from build123d import *

# Parameters (mm, degrees)
BASES_W                            = 14
BASES_H                            = 14
BASE_DEPTH                         = 14.5
NEUTRALS_W                         = 0.5
NEUTRALS_H                         = 2.8
NEUTRAL_DEPTH                      = 18.557049866
GROUNDS_W                          = 2.8
GROUNDS_H                          = 0.5
GROUND_DEPTH                       = 18.557049866
TOP_GROUND_AREA_REACH              = 23.337
SKETCH1_W                          = 2.8
SKETCH1_H                          = 11.5
SKETCH15_W                         = 2.8
SKETCH15_H                         = 12.5
GND_POCKET_EXTRA_CUT_DEPTH         = 1.75
SIDE_GROUND_AREA_DEPTH             = 5
SIDE_GND_TERMINAL_SCREW_AREA_REACH = 23.337
POCKET_START                       = -1.75
SKETCH4_W                          = 7.4
SKETCH4_H                          = 4
POCKET_GND_TERMINAL_AREA_DEPTH     = 2
SKETCH6_W                          = 12.5
SKETCH6_H                          = 3.6
NEUTRAL_SIDE_AREA_CUT_DEPTH        = 4.35
NEUTRAL_SIDE_SCREW_TERMINAL_DEPTH  = 8.4
NEUTRAL_SIDE_CURVED_WALL_CUT_REACH = 19.557
SKETCH8_W                          = 12.5
SKETCH8_H                          = 2.8
LINE_AREA_CUT_DEPTH                = 4.35
LINE_SIDE_SCREW_TERMINAL_REACH     = 23.337
SKETCH10_W                         = 7
SKETCH10_H                         = 12.3
BOTTOM_POCKET_DEPTH                = 4
SKETCH11_R                         = 2.5
FASTENER_TOP_BORE_DEPTH            = 0.5
SKETCH13_R                         = 2.35
FASTENER_BOSS_DEPTH                = 6.4
FASTENER_BOSS_TAPER                = 1
SKETCH12_R                         = 2
SKETCH14_R                         = 1.638287584


with BuildPart() as part:
    # BaseS → BASE (new body)
    with BuildSketch(Plane.XY):
        Rectangle(BASES_W, BASES_H)
    extrude(amount=BASE_DEPTH)

    # NeutralS → NEUTRAL (cut, through all)
    with BuildSketch(Plane(origin=(0, 0, 0), x_dir=(-1, 0, 0), z_dir=(0, 0, -1))):
        with Locations((4.65, 0)):
            Rectangle(NEUTRALS_W, NEUTRALS_H)
    neutral = extrude(amount=-NEUTRAL_DEPTH, mode=Mode.SUBTRACT)

    # LINE HM: NEUTRAL across plane
    add(neutral.mirror(Plane(origin=(0, 0, 0), x_dir=(0, 0, 1), z_dir=(1, 0, 0))), mode=Mode.SUBTRACT)

    # GroundS → GROUND (cut, through all)
    with BuildSketch(Plane(origin=(0, 0, 0), x_dir=(-1, 0, 0), z_dir=(0, 0, -1))):
        with Locations((0, 4.55)):
            Rectangle(GROUNDS_W, GROUNDS_H)
    extrude(amount=-GROUND_DEPTH, mode=Mode.SUBTRACT)

    # Sketch1 → TOP GROUND AREA (cut, up to next)
    with BuildSketch(Plane(origin=(0, 7, 0), x_dir=(1, 0, 0), z_dir=(0, 1, 0)), mode=Mode.PRIVATE) as top_ground_area_sk1:
        with Locations((0, -7.75)):
            Rectangle(SKETCH1_W, SKETCH1_H)
    top_ground_area_tool1 = extrude(top_ground_area_sk1.sketch, amount=-TOP_GROUND_AREA_REACH, mode=Mode.PRIVATE) & part.part
    add(top_ground_area_tool1.solids().sort_by_distance((0, 7, 7.75))[0], mode=Mode.SUBTRACT)

    # Sketch15 → GND POCKET EXTRA CUT (cut)
    with BuildSketch(Plane(origin=(0, 4.3, 0), x_dir=(1, 0, 0), z_dir=(0, 1, 0))):
        with Locations((0, -8.25)):
            Rectangle(SKETCH15_W, SKETCH15_H)
    extrude(amount=-GND_POCKET_EXTRA_CUT_DEPTH, mode=Mode.SUBTRACT)

    # Sketch2 → SIDE GROUND AREA (cut)
    with BuildSketch(Plane.XY.offset(14.5)):
        with BuildLine():
            Line((4, 7), (4, 4.05))
            ThreePointArc((4, 4.05), (3.707106781, 3.342893219), (3, 3.05))
            Line((3, 3.05), (0.6, 3.05))
            Line((0.6, 3.05), (0.6, 2.55))
            Line((0.6, 2.55), (-1.4, 2.55))
            Line((-1.4, 2.55), (-1.4, 7))
            Line((-1.4, 7), (4, 7))
        make_face()
    extrude(amount=-SIDE_GROUND_AREA_DEPTH, mode=Mode.SUBTRACT)

    # SIDE GND TERMINAL SCREW AREA: up to this face of the body (flat: up to its plane)
    side_gnd_terminal_screw_area_end = Plane(part.part.faces().sort_by_distance((1.4, 4.635, 6.044915254))[0])
    # Sketch3 → SIDE GND TERMINAL SCREW AREA (cut, up to the picked face)
    with BuildSketch(Plane(origin=(7, 0, 0), x_dir=(0, 0, -1), z_dir=(1, 0, 0)), mode=Mode.PRIVATE) as side_gnd_terminal_screw_area_sk1:
        with BuildLine():
            Line((-9.5, 9.45), (-9.5, 4.55))
            ThreePointArc((-9.5, 4.55), (-11.5, 2.55), (-13.5, 4.55))
            Line((-13.5, 4.55), (-13.5, 9.45))
            ThreePointArc((-13.5, 9.45), (-11.5, 11.45), (-9.5, 9.45))
        make_face()
    side_gnd_terminal_screw_area_tool1 = split(extrude(side_gnd_terminal_screw_area_sk1.sketch, amount=-SIDE_GND_TERMINAL_SCREW_AREA_REACH, mode=Mode.PRIVATE), bisect_by=side_gnd_terminal_screw_area_end, keep=Keep.BOTH, mode=Mode.PRIVATE)
    add(side_gnd_terminal_screw_area_tool1.solids().sort_by(Axis((7, 7, 11.5), (-1, 0, 0)))[0], mode=Mode.SUBTRACT)

    # Sketch4 → POCKET GND TERMINAL AREA (cut)
    with BuildSketch(Plane(origin=(0, 4.3, 0), x_dir=(1, 0, 0), z_dir=(0, 1, 0)).offset(POCKET_START)):
        with Locations((2.3, -11.5)):
            Rectangle(SKETCH4_W, SKETCH4_H)
    extrude(amount=POCKET_GND_TERMINAL_AREA_DEPTH, mode=Mode.SUBTRACT)

    # Sketch6 → NEUTRAL SIDE AREA CUT (cut)
    with BuildSketch(Plane.ZY.offset(7)):
        with Locations((8.25, 0.4)):
            Rectangle(SKETCH6_W, SKETCH6_H)
    extrude(amount=-NEUTRAL_SIDE_AREA_CUT_DEPTH, mode=Mode.SUBTRACT)

    # Sketch5 → NEUTRAL SIDE SCREW TERMINAL (cut)
    with BuildSketch(Plane(origin=(0, 7, 0), x_dir=(1, 0, 0), z_dir=(0, 1, 0))):
        with BuildLine():
            Line((-9.35, -9.5), (-4.65, -9.5))
            ThreePointArc((-4.65, -9.5), (-2.65, -11.5), (-4.65, -13.5))
            Line((-4.65, -13.5), (-9.35, -13.5))
            ThreePointArc((-9.35, -13.5), (-11.35, -11.5), (-9.35, -9.5))
        make_face()
    extrude(amount=-NEUTRAL_SIDE_SCREW_TERMINAL_DEPTH, mode=Mode.SUBTRACT)

    # Sketch7 → NEUTRAL SIDE CURVED WALL CUT (cut, up to next)
    with BuildSketch(Plane.XY.offset(14.5), mode=Mode.PRIVATE) as neutral_side_curved_wall_cut_sk1:
        with BuildLine():
            Line((-7, 2.2), (-2.65, 2.2))
            Line((-2.65, 2.2), (-2.65, 3))
            ThreePointArc((-2.65, 3), (-2.942893219, 3.707106781), (-3.65, 4))
            Line((-3.65, 4), (-7, 4))
            Line((-7, 4), (-7, 2.2))
        make_face()
    neutral_side_curved_wall_cut_tool1 = extrude(neutral_side_curved_wall_cut_sk1.sketch, amount=-NEUTRAL_SIDE_CURVED_WALL_CUT_REACH, mode=Mode.PRIVATE) & part.part
    add(neutral_side_curved_wall_cut_tool1.solids().sort_by_distance((-4.879997, 3.080933, 14.5))[0], mode=Mode.SUBTRACT)

    # Sketch8 → LINE AREA CUT (cut)
    with BuildSketch(Plane(origin=(7, 0, 0), x_dir=(0, 0, -1), z_dir=(1, 0, 0))):
        with Locations((-8.25, 0)):
            Rectangle(SKETCH8_W, SKETCH8_H)
    extrude(amount=-LINE_AREA_CUT_DEPTH, mode=Mode.SUBTRACT)

    # Sketch9 → LINE SIDE SCREW TERMINAL (cut, up to next)
    with BuildSketch(Plane(origin=(0, -7, 0), x_dir=(-1, 0, 0), z_dir=(0, -1, 0)), mode=Mode.PRIVATE) as line_side_screw_terminal_sk1:
        with BuildLine():
            Line((-4.65, -13.5), (-7, -13.5))
            ThreePointArc((-7, -13.5), (-9, -11.5), (-7, -9.5))
            Line((-7, -9.5), (-4.65, -9.5))
            ThreePointArc((-4.65, -9.5), (-2.65, -11.5), (-4.65, -13.5))
        make_face()
    line_side_screw_terminal_tool1 = extrude(line_side_screw_terminal_sk1.sketch, amount=-LINE_SIDE_SCREW_TERMINAL_REACH, mode=Mode.PRIVATE) & part.part
    add(line_side_screw_terminal_tool1.solids().sort_by_distance((5.825, -7, 11.5))[0], mode=Mode.SUBTRACT)

    # Sketch10 → BOTTOM POCKET (cut)
    with BuildSketch(Plane.XZ.offset(7)):
        with Locations((-1.5, 8.35)):
            Rectangle(SKETCH10_W, SKETCH10_H)
    extrude(amount=-BOTTOM_POCKET_DEPTH, mode=Mode.SUBTRACT)

    # Sketch11 → FASTENER TOP BORE (cut)
    with BuildSketch(Plane(origin=(0, 0, 0), x_dir=(-1, 0, 0), z_dir=(0, 0, -1))):
        Circle(SKETCH11_R)
    extrude(amount=-FASTENER_TOP_BORE_DEPTH, mode=Mode.SUBTRACT)

    # Sketch13 → FASTENER BOSS (add)
    with BuildSketch(Plane.XY.offset(14.5)):
        Circle(SKETCH13_R)
    extrude(amount=FASTENER_BOSS_DEPTH, taper=FASTENER_BOSS_TAPER)

    # Sketch12 → FASTENER CLEARANCE HOLE section 0
    with BuildSketch(Plane(origin=(0, 0, 0.5), x_dir=(-1, 0, 0), z_dir=(0, 0, -1))):
        Circle(SKETCH12_R)
    # Sketch14 → FASTENER CLEARANCE HOLE section 1
    with BuildSketch(Plane.XY.offset(20.9)):
        Circle(SKETCH14_R)
    loft(mode=Mode.SUBTRACT)


solid = part.part
Build history of the part. All positions in model axes, mm. A direction names the side the tool comes from. Round coordinates to 2 decimals unless told otherwise and drop trailing zeros. Order: outer loops, then holes, each group sorted by start corner. A loop starts at its lowest first (then second) coordinate and runs counter-clockwise, first axis right, second up. Notation, with made-up numbers: M -27,62 L 14,62 A29 cw 14,97 Z; hole C 51.5,43.5 d4. An arc over 180 degrees is marked long. Use CSV: the item, a comma, the result in double quotes. Start each with the question number.
(1) Cut at A-A on x = 6.25. List the corners of the cut face in (y, z), then the cut area to 3 significant figures.
(2) Flat gauge pins, fed straight in: P1, Ø0.5, axis at x = 3.5, y = 0.5, coming from the +Z side; P2, Ø4.5, axis at x = -1.5, y = -4.5, coming from the +Z side; P3, Ø1.5, axis at x = -2, z = 18, coming from the -Y side. Where does each tip first touch, or does it go through?
(3) Cut at B-B on y = -4.25. List the corners of the cut face in (x, z).
(4) Cut at C-C on z = 8.5. List the corners of the cut face in (x, y).
(5) Mould opens along X. For faces 5 (the face through (-4.4, 0, 1)), 6 (the face through (4, 0, 2)), 7 (the face through (2.65, -4.24, 11.46)) say: +X half, -X half, draft (parallel to the pull), parting line (faces both ways), or undercut.
(6) Tool access for faces 1 (the face through (6.51, 2.55, 11.46)), 2 (the face through (6, 0, 2)), 3 (the face through (0, 4.3, 1)), 4 (the face through (-2, -3, 8)): list every direction of +Z, -Z, +X, -X, +Y, -Y with a clear straight run to the whole face (end or side of a thin tool).
(7) Drill centre lines: probe 1 along Y at (x, z) = (0, 0.35); probe 2 along Z at (x, y) = (4.75, 4.75); probe 3 along Y at (x, z) = (3, 6.25). Where is each one in solid material? Low to high.
(8) Cut at D-D on x = -4. List the corners of the cut face in (y, z).
Findings:
1,outline,"M -7,0 L 7,0 L 7,9.5 L 4.55,9.5 A2 cw 4.55,13.5 L 7,13.5 L 7,14.5 L 1.4,14.5 L 1.4,2 L -1.4,2 L -1.4,9.5 L -7,9.5 Z; M -7,13.5 L -1.4,13.5 L -1.4,14.5 L -7,14.5 Z"
1,area,"130 mm^2"
2,P1,"stops at z = 2"
2,P2,"stops at z = 14.5"
2,P3,"stops at y = -1.92"
3,outline,"M -7,0 L 7,0 L 7,9.5 L 4.65,9.5 A2 cw 4.65,13.5 L 7,13.5 L 7,14.5 L 2,14.5 L 2,2.2 L -5,2.2 L -5,14.5 L -7,14.5 Z"
4,outline,"M -7,-7 L -5,-7 L -5,-3 L 2,-3 L 2,-7 L 7,-7 L 7,-1.4 L 2.65,-1.4 L 2.65,1.4 L 7,1.4 L 7,7 L 1.4,7 L 1.4,2.55 L -1.4,2.55 L -1.4,7 L -7,7 L -7,2.2 L -2.65,2.2 L -2.65,-1.4 L -7,-1.4 Z; hole C 0,0 d3.72"
5,face 5,"undercut"
5,face 6,"draft"
5,face 7,"+X half"
6,face 1,"+X, +Y"
6,face 2,"+Z, +X"
6,face 3,"+Z, -Z"
6,face 4,"+Z, -Y"
7,probe 1,"y = -7 to -2.5, 2.5 to 4.3, 4.8 to 7"
7,probe 2,"z = 0 to 9.5, 13.5 to 14.5"
7,probe 3,"y = -7 to -1.4, 1.4 to 7"
8,outline,"M -7,0 L 7,0 L 7,9.61 L 2.2,9.61 L 2.2,2 L -1.4,2 L -1.4,14.5 L -3,14.5 L -3,2.2 L -7,2.2 Z; M 4,13.39 L 7,13.39 L 7,14.5 L 4,14.5 Z"
